Read the model definition and answer for the solid it produces. Units are mm, in the model's axes. Face numbers are marked on the shaded views. A direction names the side the tool comes from. Coordinates: 2 decimals unless noted, no trailing zeros. Order: outer loops, then holes, each group sorted by start corner. A loop starts at its lowest first (then second) coordinate and runs counter-clockwise, first axis right, second up. Notation, with made-up numbers: M -6.75,77 L 18.25,77 A14 ccw 18.25,88 Z; hole C 76.25,-8 d11. An arc over 180 degrees is marked long. Put each result on its own line as item: value.
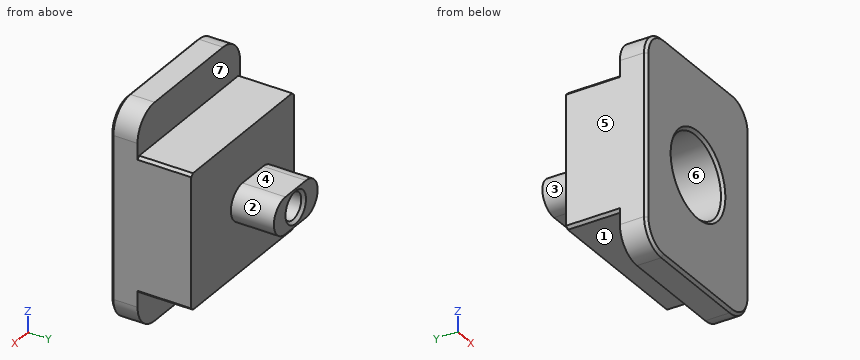
Autodesk Inventor part; units mm, degrees
ref_plane "YZ Plane" through (0, 0, 0) normal (1, 0, 0) x (0, 1, 0)
ref_plane "XZ Plane" through (0, 0, 0) normal (0, 1, 0) x (-1, 0, 0)
ref_plane "XY Plane" through (0, 0, 0) normal (0, 0, 1) x (1, 0, 0)
sketch "Sketch1" plane through (0, 0, 0) normal (0, 1, 0) x (-1, 0, 0)
  line L0 (15, 20) -> (-15, 20)
  line L1 (-15, 20) -> (-15, -20)
  line L2 (-15, -20) -> (15, -20)
  line L3 (15, -20) -> (15, 20)
  line L4 (15, 20) -> (-15, -20) construction
  line L5 (-15, 20) -> (15, -20) construction
  line L6 (21, 0) -> (-21, 0) construction
  line L7 (0, -28) -> (0, 28) construction
  line L8 (6, 0) -> (0, 0) construction
  line L9 (6, 3.4) -> (0, 3.4)
  line L10 (0, -3.4) -> (6, -3.4)
  arc A0 (6, -3.4) -> (6, 3.4) centre (6, 0) ccw
  arc A1 (0, 3.4) -> (0, -3.4) centre (0, 0) ccw
  line L11 (-15, 12.5) -> (15, 12.5)
  line L12 (-15, -12.5) -> (15, -12.5)
  point P0 (0, 0)
  point P1 (3, 0)
  point P2 (3, 0)
  point P3 (15, -12.5)
  dimension "d0" = 40
  dimension "d1" = 30
  dimension "d2" = 6
  dimension "d3" = 6.8
  dimension "d19" = 3
  dimension "d35" = 25
extrude "Extrusion1" add sketch "Sketch1" against normal blind 23 contours L3 L11 L1 L0 | L3 L12 L1 L11 | L3 L2 L1 L12 | A0 L10 A1 L9
extrude "Extrusion2" cut sketch "Sketch1" against normal blind 8
sketch "Sketch3" plane through (0, -23, 0) normal (0, -1, 0) x (1, 0, 0)
  circle A0 centre (0, 0) radius 7.5
  dimension "d29" = 15
extrude "Extrusion5" cut sketch "Sketch3" against normal blind 10
extrude "Extrusion6" cut sketch "Sketch1" against normal blind 18 contours L3 L11 L1 L0 | L3 L2 L1 L12
hole "Hole1" at (-3, 0, 0) direction (0, -1, 0) diameter 4.917 depth 13 countersink diameter 6 countersink angle 90
fillet "Fillet1" radius 5 4 edges at (-15, -20.5, 20) (-15, -20.5, -20) (15, -20.5, -20) (15, -20.5, 20)
chamfer "Chamfer1" distance 0.5 angle 45 13 edges at (0, -23, 20) (-13.5355, -23, 18.5355) (-15, -23, 0) (-13.5355, -23, -18.5355) (0, -23, -20) (13.5355, -23, -18.5355) (15, -23, 0) (13.5355, -23, 18.5355) (-7.5, -23, 0) (-15, -13, 12.5) (-15, -13, -12.5) (15, -13, -12.5) (15, -13, 12.5)
equation "\"d4\" = slotTabH + sheetT"
equation "\"d6\" = slotTabH"
equation "\"slotTabH\" = 8"
equation "\"sheetT\" = 15"
equation "\"totalHeight\" = slotTabH + sheetT"
properties part number "TCSM1-X-003" material "Steel"
Q1. Find section B-B on y = -16.5. Write down the section's boundary in (x, z).
Answers below:
outline: M -15,-12 L -14.5,-12.5 L 14.5,-12.5 L 15,-12 L 15,12 L 14.5,12.5 L -14.5,12.5 L -15,12 Z; hole C 0,0 d15
Q2. Find section A-A on z = 0. Write down the section's boundary in (x, y).
Answers below:
outline: M -15,-22.5 L -14.5,-23 L -8,-23 L -7.5,-22.5 L -7.5,-13 L -5.46,-13 L -5.46,-0.54 L -6,0 L -9.4,0 L -9.4,-8 L -15,-8 Z; M -0.54,-13 L 7.5,-13 L 7.5,-22.5 L 8,-23 L 14.5,-23 L 15,-22.5 L 15,-8 L 3.4,-8 L 3.4,0 L 0,0 L -0.54,-0.54 Z
Q3. A tool of negligible diameter and unlimited length cuts with its end or side. For the marked faces 1, 2, 3 and 4, from which of +Z, -Z, +X, -X, +Y, -Y can it reach the whole face along a straight path? Write none if from no direction.
Answers below:
face 1: -Z, +X, -X, +Y
face 2: +X, +Y
face 3: -X, +Y
face 4: +Z, +X, -X, +Y
Q4. For a pull along X with two mould halves and no side action, classify the marked faces 5, 6 and 7 as +X half, -X half, draft (parallel to the pull), parting line (faces both ways), or undercut.
Answers below:
face 5: -X half
face 6: undercut
face 7: draft
Q5. Find section D-D on y = -11.75. Write down the section's boundary in (x, z), plus the area to 3 significant figures.
Answers below:
outline: M -15,-12 L -14.5,-12.5 L 14.5,-12.5 L 15,-12 L 15,12 L 14.5,12.5 L -14.5,12.5 L -15,12 Z; hole C -3,0 d4.92
area: 731 mm^2
Q6. Given pin 1 (3 mm diameter, centred on x = -2.5, y = -6, fed in from +Z); pin 2 (10 mm diameter, centred on x = 7, y = -12.5, fed in from +Z); pin 3 (5 mm diameter, centred on x = 11, z = 14.5, fed in from +Y), each flat-ended and moving along its own axis, determine where each tip first touches the part or whether it passes through.
Answers below:
pin 1: stops at z = 3.4
pin 2: stops at z = 12.5
pin 3: stops at y = -8
Q7. Consider line 1 along Z through (x, y) = (-3, -5.75); line 2 along Z through (x, y) = (0, -19); line 3 along Z through (x, y) = (4.5, -8.25). Determine where each line is inside the solid, lowest interval first.
Answers below:
line 1: z = -3.4 to -2.46, 2.46 to 3.4
line 2: z = -20 to -7.5, 7.5 to 20
line 3: z = -12.5 to 12.5
Q8. Find section C-C on z = -10. Write down the section's boundary in (x, y).
Answers below:
outline: M -15,-22.5 L -14.5,-23 L 14.5,-23 L 15,-22.5 L 15,-8 L -15,-8 Z
